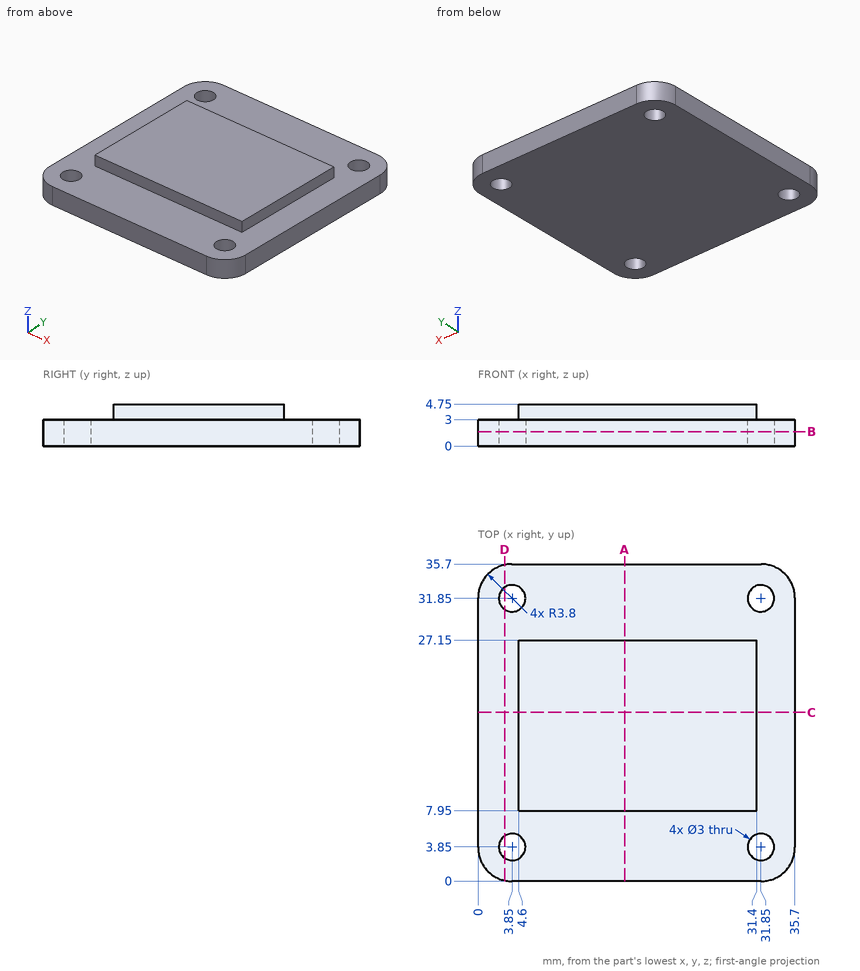
Source: three-view drawing plus pictorial views. Frame: mm from the lowest corner of the part. Coordinates: 2 decimals unless noted, no trailing zeros. Order: outer loops, then holes, each group sorted by start corner. A loop starts at its lowest first (then second) coordinate and runs counter-clockwise, first axis right, second up. Notation, with made-up numbers: M 17,51.5 L 54,51.5 A34 cw 54,84.5 Z; hole C -29.5,6 d3. An arc over 180 degrees is marked long. Answer in a Markdown table with one row per item.
(1) Section query B-B, the plane z = 1.65. Output: boundary loops of the cut face in (x, y).
Numbers:
| item | result |
|---|---|
| outline | M 0,3.8 A3.8 ccw 3.8,0 L 31.9,0 A3.8 ccw 35.7,3.8 L 35.7,31.9 A3.8 ccw 31.9,35.7 L 3.8,35.7 A3.8 ccw 0,31.9 Z; hole C 3.85,3.85 d3; hole C 3.85,31.85 d3; hole C 31.85,3.85 d3; hole C 31.85,31.85 d3 |
(2) Contact query for flat-ended pins moving along their axis: pin 1 Ø1.9 at (y, z) = (20.5, 4.5) entering from +X; pin 2 Ø0.5 at (y, z) = (13.5, 4) entering from -X; pin 3 Ø2 at (x, y) = (28.5, 30) entering from +Z. Output: stop coordinate, or through.
Numbers:
| item | result |
|---|---|
| pin 1 | stops at x = 31.4 |
| pin 2 | stops at x = 4.6 |
| pin 3 | stops at z = 3 |
(3) Material intervals for line 1 (Y direction, x = 3.85, z = 1.75); line 2 (Y direction, x = 5, z = 0.6); line 3 (Z direction, x = 22, y = 31.5), sorted ascending. Write a range as [from, to].
Numbers:
| item | result |
|---|---|
| line 1 | y = [0, 2.35], [5.35, 30.35], [33.35, 35.7] |
| line 2 | y = [0, 2.89], [4.81, 30.89], [32.81, 35.7] |
| line 3 | z = [0, 3] |
(4) Section query D-D, the plane x = 3. Output: boundary loops of the cut face in (y, z), plus the area to 3 significant figures.
Numbers:
| item | result |
|---|---|
| outline | M 0.09,0 L 2.61,0 L 2.61,3 L 0.09,3 Z; M 5.09,0 L 30.61,0 L 30.61,3 L 5.09,3 Z; M 33.09,0 L 35.61,0 L 35.61,3 L 33.09,3 Z |
| area | 91.8 mm^2 |
(5) Section query C-C, the plane y = 19. Output: boundary loops of the cut face in (x, z), plus the area to 3 significant figures.
Numbers:
| item | result |
|---|---|
| outline | M 0,0 L 35.7,0 L 35.7,3 L 31.4,3 L 31.4,4.75 L 4.6,4.75 L 4.6,3 L 0,3 Z |
| area | 154 mm^2 |
(6) Section query A-A, the plane x = 16.5. Output: boundary loops of the cut face in (y, z).
Numbers:
| item | result |
|---|---|
| outline | M 0,0 L 35.7,0 L 35.7,3 L 27.15,3 L 27.15,4.75 L 7.95,4.75 L 7.95,3 L 0,3 Z |
